Could you check a few things on this model? Use its own coordinates, in mm. A direction names the side the tool comes from. Coordinates: 2 decimals unless noted, no trailing zeros. Write each loop counter-clockwise with the first axis right and the second up, starting at its lowest first coordinate (ties: lowest second). Pieces come first, ordered by that corner, then holes. Notation, with made-up numbers: (42.25, -4.5) - (62.25, -4.5) arc R14 cw to (62.25, 12.5) - close; hole circle Ø5 at (-25, -26). An arc over 180 degrees is marked (long way). Answer as a JSON object with one key per item and string values. Group by question number.
1) If we section it at B-B (y = 4.5): Write out the boundary of the cut face in (x, z) (3 decimals).
2) Please list where these lines run through material, in increasing order: line 1 along Z through (x, y) = (0, 2.4); line 2 along Y through (x, z) = (-0.95, 0.5).
3) We'd pull the mould along X, two halves only. Please class faces 1 (the flat face through (1, 6, 0.895)), 2 (the flat face through (-0.895, 6, 2)), 3 (the flat face through (0.655, 6, 2)), 4 (the cylindrical face through (1.27, 1.48, 0.97)): released by +X, released by -X, zero draft, split by the parting line, or undercut.
4) Will these pins go through, and if not, where does the flat tip stop? pin 1 Ø1 at (x, z) = (-0.5, -0.5) entering from -Y; pin 2 Ø1.2 at (y, z) = (7, 2) entering from +X (3 decimals); pin 3 Ø1.5 at (y, z) = (4.5, 2) entering from +X.
5) On a 3-axis mill with a long thin cutter (end or side, diameter ignored), from which of +Z, -Z, +X, -X, +Y, -Y can I reach the whole of each face in a straight line? I mean faces 5 (the flat face through (-2, 6, 0.895)), 6 (the flat face through (1.1, 4, 1.3)), 7 (the flat face through (-0.895, 6, -1)), 8 (the flat face through (0.655, 6, -1)). Say none if no direction works.
6) If we section it at C-C (x = -1.8): Write out the boundary of the cut face in (y, z) (3 decimals).
```python
from build123d import *

# Parameters (mm, degrees)
SKETCH1_R           = 2.1
BOSS_EXTRUDE1_DEPTH = 4
SKETCH2_R           = 1.6
CUT_EXTRUDE1_DEPTH  = 3
BOSS_EXTRUDE2_DEPTH = 5


with BuildPart() as part:
    # Sketch1 → Boss-Extrude1 (new body)
    with BuildSketch(Plane(origin=(0, 0, 0), x_dir=(1, 0, 0), z_dir=(0, 1, 0))):
        Circle(SKETCH1_R)
    extrude(amount=BOSS_EXTRUDE1_DEPTH)

    # Sketch2 → Cut-Extrude1 (cut)
    with BuildSketch(Plane(origin=(0, 0, 0), x_dir=(-1, 0, 0), z_dir=(0, -1, 0))):
        Circle(SKETCH2_R)
    extrude(amount=-CUT_EXTRUDE1_DEPTH, mode=Mode.SUBTRACT)

    # Sketch3 → Boss-Extrude2 (add)
    with BuildSketch(Plane(origin=(0, 4, 0), x_dir=(1, 0, 0), z_dir=(0, 1, 0))):
        Polygon((-0.895, 0.655), (-2.39, 0.655), (-2.39, -0.895), (-0.895, -0.895), (-0.895, -2.39), (0.655, -2.39), (0.655, -0.895), (2.11, -0.895), (2.11, 0.655), (0.655, 0.655), (0.655, 2.11), (-0.895, 2.11), align=None)
    extrude(amount=BOSS_EXTRUDE2_DEPTH)


solid = part.part
```
Here are the results:
{
 "1": {"outline": "(-2.39, -0.655) - (-0.895, -0.655) - (-0.895, -2.11) - (0.655, -2.11) - (0.655, -0.655) - (2.11, -0.655) - (2.11, 0.895) - (0.655, 0.895) - (0.655, 2.39) - (-0.895, 2.39) - (-0.895, 0.895) - (-2.39, 0.895) - close"},
 "2": {"line 1": "z = -2.1 to -1.6, 1.6 to 2.1", "line 2": "y = 3 to 9"},
 "3": {"face 1": "zero draft", "face 2": "released by -X", "face 3": "released by +X", "face 4": "undercut"},
 "4": {"pin 1": "stops at y = 3", "pin 2": "stops at x = 0.655", "pin 3": "stops at x = 1.53"},
 "5": {"face 5": "+Z, -X, +Y", "face 6": "+Z, +X, +Y", "face 7": "-Z, -X, +Y", "face 8": "-Z, +X, +Y"},
 "6": {"outline": "(0, -1.082) - (4, -1.082) - (4, -0.655) - (9, -0.655) - (9, 0.895) - (4, 0.895) - (4, 1.082) - (0, 1.082) - close"}
}
